Geometry check sheet. Reference: the model listing, model coordinates, mm. Face numbers are marked on the shaded views. A direction names the side the tool comes from. Round coordinates to 2 decimals unless told otherwise and drop trailing zeros. Write each loop counter-clockwise with the first axis right and the second up, starting at its lowest first coordinate (ties: lowest second). Pieces come first, ordered by that corner, then holes. Notation, with made-up numbers: (34, 14) -> (43, 14) arc R30 cw to (43, 41) -> close; hole circle Ø11 at (-39, -19). An arc over 180 degrees is marked (long way). Use a Markdown table: item, result.
```python
from build123d import *

# Parameters (mm, degrees)
SKETCH1_W           = 6
SKETCH1_H           = 6
BOSS_EXTRUDE1_DEPTH = 5
CUT_EXTRUDE4_DEPTH  = 12.5
CUT_EXTRUDE5_DEPTH  = 2.5


with BuildPart() as part:
    # Sketch1 → Boss-Extrude1 (new body)
    with BuildSketch(Plane(origin=(0, 0, 0), x_dir=(1, 0, 0), z_dir=(0, 1, 0))):
        Rectangle(SKETCH1_W, SKETCH1_H)
    extrude(amount=BOSS_EXTRUDE1_DEPTH)

    # Sketch5 → Cut-Extrude4 (cut)
    with BuildSketch(Plane.XY.offset(3)):
        with BuildLine():
            Line((-3, 5), (-3, 2.5))
            ThreePointArc((-3, 2.5), (-1.952562419, 4.293074903), (0, 5))
            Line((0, 5), (-3, 5))
        make_face()
        with BuildLine():
            ThreePointArc((0, 5), (1.952562419, 4.293074903), (3, 2.5))
            Line((3, 2.5), (3, 5))
            Line((3, 5), (0, 5))
        make_face()
        with BuildLine():
            ThreePointArc((-3, 0), (0, 2), (3, 0))
            Line((3, 0), (-3, 0))
        make_face()
    extrude(amount=-CUT_EXTRUDE4_DEPTH, mode=Mode.SUBTRACT)

    # Sketch6 → Cut-Extrude5 (cut)
    with BuildSketch(Plane.XY.offset(3)):
        with BuildLine():
            Line((-3, 2.5), (-3, 2))
            Line((-3, 2), (0, 5))
            ThreePointArc((0, 5), (-1.952562419, 4.293074903), (-3, 2.5))
        make_face()
        with BuildLine():
            Line((0, 2), (-3, 2))
            Line((-3, 2), (-3, 0))
            ThreePointArc((-3, 0), (-1.802775638, 1.454163457), (0, 2))
        make_face()
    extrude(amount=-CUT_EXTRUDE5_DEPTH, mode=Mode.SUBTRACT)


solid = part.part
```
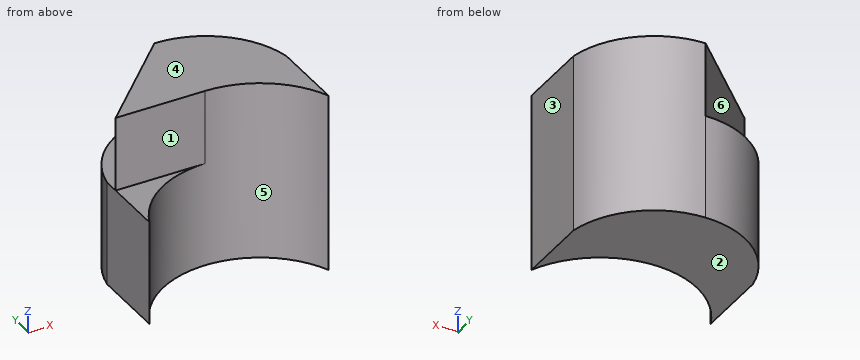
(1) Access from +Z, -Z, +X, -X, +Y, -Y to the whole of each face (thin tool, end or side, straight path). Record for the marked faces 1 and 2.
A:
| item | result |
|---|---|
| face 1 | +Z, -X, -Y |
| face 2 | -Z, +X, -X, +Y, -Y |
(2) Section check B-B on y = 2.4. Record the cut outline in (x, z).
A:
| item | result |
|---|---|
| outline | (-3, -3) -> (3, -3) -> (3, 3) -> (-2.6, 3) -> (-2.6, 0.5) -> (-3, 0.5) -> close |
(3) Section check D-D on z = 2.05. Record the cut outline in (x, y), plus the area to 3 significant figures.
A:
| item | result |
|---|---|
| outline | (-3, 2) -> (0, 2) arc R3.25 cw to (3, 0) -> (3, 2.5) arc R3.05 ccw to (0, 5) -> close |
| area | 13.3 mm2 |
(4) Section check C-C on x = -1.75. Record the cut outline in (y, z), plus the area to 3 significant figures.
A:
| item | result |
|---|---|
| outline | (1.49, -3) -> (4.45, -3) -> (4.45, 0.5) -> (3.25, 0.5) -> (3.25, 3) -> (2, 3) -> (2, 0.5) -> (1.49, 0.5) -> close |
| area | 13.5 mm2 |
(5) Section check A-A on y = 1.8. Record the cut outline in (x, z).
A:
| item | result |
|---|---|
| outline | (-3, -3) -> (-1.12, -3) -> (-1.12, 0.5) -> (-3, 0.5) -> close; (1.12, -3) -> (3, -3) -> (3, 3) -> (1.12, 3) -> close |
(6) Gauge pin test, flat end, axial feed: pin 1 Ø1.2 at (x, z) = (-1.5, 2.5) entering from -Y. Record the tip position at first contact, or that the pin passes through.
A:
| item | result |
|---|---|
| pin 1 | stops at y = 2 |
(7) Release check for a two-part mould opening along X. For the marked faces 3, 4, 5 and 6 record: +X half, -X half, draft (parallel to the pull), parting line (faces both ways), or undercut.
A:
| item | result |
|---|---|
| face 3 | +X half |
| face 4 | draft |
| face 5 | undercut |
| face 6 | -X half |
(8) Thickness scan on line 1 (X direction, y = 1.3, z = -0.65); line 2 (X direction, y = 4.75, z = 0.4); line 3 (X direction, y = 2.8, z = -0.45). Record the ranges inside material, lowest first.
A:
| item | result |
|---|---|
| line 1 | x = -3 to -2.01, 2.01 to 3 |
| line 2 | x = -1.21 to 1.21 |
| line 3 | x = -2.93 to 2.93 |
